```python
from build123d import *

# Parameters (mm, degrees)
F0_R          = 12.55
F0_R_2        = 10.9
F0_R_3        = 3.25
F0_R_4        = 5.1
F0_R_5        = 2.5
F1_DEPTH      = 9
F2_DEPTH      = 10
F3_R          = 10
F4_R          = 5
F11_DEPTH     = 2.9
F10_R         = 3.25
F13_T4_ANGLE  = 230.6618088311
F13_S5_R      = 3.25
F13_T6_DEPTH  = 6
F13_T10_ANGLE = 171.9012593912
F13_S11_R     = 3.25
F13_T12_DEPTH = 5


# Not quite as in the source:
# - a fillet or chamfer that OpenCascade refuses, or shapes differently, is made with other operations: its cross-section is extruded or revolved along the edge and cut away or added


with BuildPart() as f1:
    # F0 (on Right) → F1 (new body)
    with BuildSketch(Plane.YZ):
        with BuildLine():
            Line((7.45, 25.2829590551), (-23.7829060836, 25.2829590551))
            ThreePointArc((-23.7829060836, 25.2829590551), (-39.2686382031, 4.2232189691), (-14.55, -4.280278967))
            Line((-14.55, -4.280278967), (-14.55, -14.55))
            Line((-14.55, -14.55), (14.55, -14.55))
            Line((14.55, -14.55), (14.55, 18.1829590551))
            ThreePointArc((14.55, 18.1829590551), (12.4704581464, 23.2034172015), (7.45, 25.2829590551))
        make_face()
        Circle(F0_R, mode=Mode.SUBTRACT)
        with Locations((-23.7829060836, 9.059573843)):
            Circle(F0_R_2, mode=Mode.SUBTRACT)
        with Locations((-7.9205860656, 17.9829590551)):
            Circle(F0_R_3, mode=Mode.SUBTRACT)
        with Locations((7.45, 18.1829590551)):
            Circle(F0_R_4, mode=Mode.SUBTRACT)
        with Locations((-7.9205860656, 17.9829590551)):
            Circle(F0_R_3)
        with Locations((-7.9205860656, 17.9829590551)):
            Circle(F0_R_5, mode=Mode.SUBTRACT)
    extrude(amount=F1_DEPTH)

    # F0 (on Right) → F2 (join)
    with BuildSketch(Plane.YZ):
        with BuildLine():
            Line((7.45, 25.2829590551), (-23.7829060836, 25.2829590551))
            ThreePointArc((-23.7829060836, 25.2829590551), (-39.2686382031, 4.2232189691), (-14.55, -4.280278967))
            Line((-14.55, -4.280278967), (-14.55, -14.55))
            Line((-14.55, -14.55), (14.55, -14.55))
            Line((14.55, -14.55), (14.55, 18.1829590551))
            ThreePointArc((14.55, 18.1829590551), (12.4704581464, 23.2034172015), (7.45, 25.2829590551))
        make_face()
        Circle(F0_R, mode=Mode.SUBTRACT)
        with Locations((-23.7829060836, 9.059573843)):
            Circle(F0_R_2, mode=Mode.SUBTRACT)
        with Locations((-7.9205860656, 17.9829590551)):
            Circle(F0_R_3, mode=Mode.SUBTRACT)
        with Locations((7.45, 18.1829590551)):
            Circle(F0_R_4, mode=Mode.SUBTRACT)
        with Locations((-23.7829060836, 9.059573843)):
            Circle(F0_R_2)
    extrude(amount=-F2_DEPTH)

    # F3
    f3_edges = [f1.edges().sort_by_distance(p)[0] for p in [
        (-0.5, -23.782906, 25.282959),
        (-0.5, 14.55, 18.182959),
        (-0.5, 7.45, 25.282959),
        (-0.5, -14.55, -14.55),
        (-0.5, 14.55, -14.55),
    ]]
    fillet(f3_edges, radius=F3_R)

    # F4
    f4_edges = [f1.edges().sort_by_distance(p)[0] for p in [
        (-0.5, -14.55, -4.280279),
    ]]
    fillet(f4_edges, radius=F4_R)

    # F7 (on plane+point) → F8 (revolve)
    with BuildSketch(Plane.XY.offset(9.059573843)):
        Polygon((1, -12.7829060836), (0, -12.7829060836), (0, -20.5329060836), (4.5, -20.5329060836), (4.5, -20.078861435), (3, -19.5329060836), (1, -19.5329060836), align=None)
    revolve(axis=Axis((4.5, -23.7829060836, 9.059573843), (1, 0, 0)))

    # F0 (on Right) → F11 (join)
    with BuildSketch(Plane.YZ):
        with Locations((-7.9205860656, 17.9829590551)):
            Circle(F0_R_3)
        with Locations((-7.9205860656, 17.9829590551)):
            Circle(F0_R_5, mode=Mode.SUBTRACT)
    extrude(amount=-F11_DEPTH)

    # F12: sweep along a path in F9
    with BuildLine(Plane(origin=(0, -9.5885144747, 17.044662029), x_dir=(1, 0, 0), z_dir=(0, 0.4902958908, -0.8715560449))) as f12_path:
        ThreePointArc((0, 16.2862637363), (-4.2426406871, 14.5289044234), (-6, 10.2862637363))
        Line((-6, 10.2862637363), (-6, -1.9137362637))
    # F10 (on face) → F12 (sweep, cut)
    with BuildSketch(Plane.YZ):
        with Locations((-23.7829060836, 9.059573843)):
            Circle(F10_R)
    sweep(path=f12_path.line, mode=Mode.SUBTRACT)

    # F13: chamfer of 0.75 on 1 edges, made by hand


with BuildPart() as f13_tool2:
    # F13_s3 → F13_t4 (revolve)
    with BuildSketch(Plane.XY.offset(17.9829590551)):
        Polygon((-2.9, -4.6705860656), (-2.15, -5.4205860656), (-2.9, -5.4205860656), align=None)
    revolve(axis=Axis((-2.9, -7.9205860656, 17.9829590551), (1, 0, 0)), revolution_arc=F13_T4_ANGLE)

    # F13_s5 → F13_t6 (intersect, symmetric)
    with BuildSketch(Plane.YZ.offset(-2.5)):
        with Locations((-7.9205860656, 17.9829590551)):
            Circle(F13_S5_R)
    extrude(amount=F13_T6_DEPTH, both=True, mode=Mode.INTERSECT)


with BuildPart() as f1_1:
    add(f1.part)

    # F13_t1: cut F13_tool2
    add(f13_tool2.part, mode=Mode.SUBTRACT)


with BuildPart() as f13_tool8:
    # F13_s9 → F13_t10 (revolve)
    with BuildSketch(Plane(origin=(0, -2.6653633076, 18.7307701592), x_dir=(1, 0, 0), z_dir=(0, -0.1408794707, 0.9900267546))):
        Polygon((-2.9, -8.558162364), (-2.15, -7.808162364), (-2.9, -7.808162364), align=None)
    revolve(axis=Axis((-2.9, -7.9205860656, 17.9829590551), (1, 0, 0)), revolution_arc=F13_T10_ANGLE)

    # F13_s11 → F13_t12 (intersect, symmetric)
    with BuildSketch(Plane.YZ.offset(-2.5)):
        with Locations((-7.9205860656, 17.9829590551)):
            Circle(F13_S11_R)
    extrude(amount=F13_T12_DEPTH, both=True, mode=Mode.INTERSECT)


with BuildPart() as f1_2:
    add(f1_1.part)

    # F13_t7: cut F13_tool8
    add(f13_tool8.part, mode=Mode.SUBTRACT)


solid = f1_2.part
```
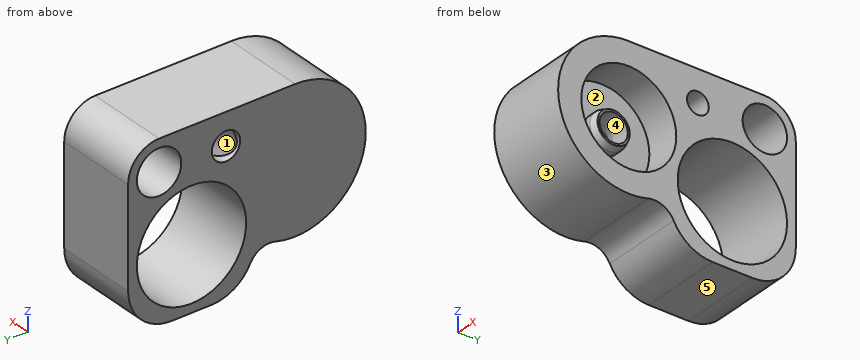
Work out the finished part from the listing and answer in its coordinate system (mm). Face numbers are marked on the shaded views. A direction names the side the tool comes from. Give positions to 0.01 mm unless a question says otherwise; leave off trailing zeros. Loops run counter-clockwise (first coordinate to the right, second up) from the corner with the lowest first, then second, coordinate; pieces in that order, holes last. Notation, with made-up numbers: (18, 7) - (26, 7) arc R28 ccw to (26, 38) - close; hole circle Ø11 at (36, -1.75). An arc over 180 degrees is marked (long way). Use CSV: the item, a comma, the result in double quotes. Start each with the question number.
(1) Find section A-A, the plane y = 0. Determine the outline of the cut face in (x, z).
(2) Find section C-C, the plane y = -33. Determine the outline of the cut face in (x, z).
(3) A tool of negligible diameter and unlimited length cuts with its end or side. For the marked faces 4 and 5, from which of +Z, -Z, +X, -X, +Y, -Y can it reach the whole face along a straight path? Write none if from no direction.
(4) Find the intervals of material crossed by L1, parallel to Y at x = -6.25, z = 18; L2, parallel to Z at x = -1.5, y = 5; L3, parallel to Y at x = -2.25, z = 8, in increasing order.
(5) Determine the mould class of the marked faces 1, 2 and 3 for opening direction X: released by +X, released by -X, zero draft, split by the parting line, or undercut.
(6) Find section B-B, the plane z = 3.5. Determine the outline of the cut face in (x, y), plus the area to 3 significant figures.
(7) Each of these flat-tipped pins is pushed along its axis until it touches: pin 1 (13 mm diameter, centred on y = -23.78, z = 9.06, fed in from +X); pin 2 (6 mm diameter, centred on y = -7.92, z = 17.98, fed in from -X); pin 3 (3.5 mm diameter, centred on y = -23.5, z = 10, fed in from +X); pin 4 (15 mm diameter, centred on y = 0, z = 0, fed in from -X). Where does it stop, or does it pass through?
(8) Find section D-D, the plane x = 7.5. Count the separate pieces of the cut face and the enclosed holes in it, plus the area to 3 significant figures.
Results found:
1,outline,"(-10, -14.55) - (9, -14.55) - (9, -12.55) - (-10, -12.55) - close; (-10, 12.55) - (9, 12.55) - (9, 25.28) - (-10, 25.28) - close"
2,outline,"(-10, -4.29) - (9, -4.29) - (9, 3.24) - (1, 3.24) - (1, 14.88) - (9, 14.88) - (9, 22.41) - (-10, 22.41) - close"
3,face 4,"+X"
3,face 5,"-Z, +X, -X, +Y, -Y"
4,L1,"-37.32 to -14.5, -4.67 to 2.35, 12.55 to 14.55"
4,L2,"-14.54 to -11.51, 11.51 to 13.71, 22.66 to 25.28"
4,L3,"-39.97 to -26.56, -20.26 to -9.67, 9.67 to 14.55"
5,face 1,"undercut"
5,face 2,"released by +X"
5,face 3,"zero draft"
6,outline,"(-10, -39.02) - (9, -39.02) - (9, -33.16) - (1, -33.16) - (1, -14.41) - (9, -14.41) - (9, -12.05) - (-10, -12.05) - close; (-10, 12.05) - (9, 12.05) - (9, 14.55) - (-10, 14.55) - close"
6,area,"410 mm^2"
7,pin 1,"x = 4.5"
7,pin 2,"x = -2.65"
7,pin 3,"x = -5.63"
7,pin 4,"through"
8,separate pieces,"1"
8,enclosed holes,"4"
8,area,"846 mm^2"
